Part model, mm, in its own coordinate system. A direction names the side the tool comes from. Coordinates: 2 decimals unless noted, no trailing zeros. Loops run counter-clockwise (first coordinate to the right, second up) from the corner with the lowest first, then second, coordinate; pieces in that order, holes last. Notation, with made-up numbers: (-25.75, -36.75) -> (29.25, -36.75) arc R12 cw to (29.25, -16.75) -> close; hole circle Ø2 at (-10, 1). An arc over 180 degrees is marked (long way). One line per question, with ' | ' between items. Start each with the question number.
1) 3-axis set-ups, long thin cutter, end or side, ignore diameter. For faces 1 (the face through (104.514, 32.972, -17.15)), 2 (the face through (-12, 0, 4)), 3 (the face through (4, -21, 21)): which of +Z, -Z, +X, -X, +Y, -Y reach the whole face in a straight line?
2) Cut at B-B (y = 0). List the corners of the cut face in (x, z).
3) Probe L1, parallel to X at y = 18.5, z = -14; L2, parallel to X at y = -44.5, z = -15; L3, parallel to Y at x = 5.5, z = 15.5. List the from-to ranges inside material, lowest first. Write a range as from..to.
4) Two-plate mould, pull along Z, no slides. Class faces 4 (the face through (-20, 0, 0)), 5 (the face through (4, -21, -21)), 6 (the face through (48.86, 2.64, 59.94)): released by +Z, released by -Z, zero draft, split by the parting line, or undercut.
5) Cut at A-A (z = 0). List the corners of the cut face in (x, y), plus the area to 3 significant figures.
6) Drop flat-ended pins along their axis: pin 1 (1.3 mm diameter, centred on y = -20.5, z = 21, fed in from -X); pin 2 (1.8 mm diameter, centred on x = -11.5, z = 4.5, fed in from +Y); pin 3 (1.6 mm diameter, centred on y = 0, z = 5, fed in from -X). Give the stop position or say it passes through.
7) Cut at C-C (x = 7.5). List the corners of the cut face in (y, z), plus the area to 3 significant figures.
from build123d import *

# Parameters (mm, degrees)
BOSS_EXTRUDE1_START = 4
SKETCH1_R           = 60
BOSS_EXTRUDE1_DEPTH = 91
SKETCH3_R           = 47.5
SKETCH3_R_2         = 2.25
BOSS_EXTRUDE2_DEPTH = 4
SKETCH4_R           = 6
BOSS_EXTRUDE3_DEPTH = 20
CUT_EXTRUDE1_START  = -15
CUT_EXTRUDE1_DEPTH  = 15


with BuildPart() as part:
    # Sketch1 → Boss-Extrude1 (new body)
    with BuildSketch(Plane(origin=(0, 0, 0), x_dir=(0, 0, -1), z_dir=(1, 0, 0)).offset(BOSS_EXTRUDE1_START)):
        Circle(SKETCH1_R)
    extrude(amount=BOSS_EXTRUDE1_DEPTH)

    # Sketch2 → Revolve1 (revolve)
    with BuildSketch(Plane.XY, mode=Mode.PRIVATE) as revolve1_sk:
        Polygon((95, 60), (105, 36), (105, 11), (109, 11), (109, 0), (105, 0), (95, 0), align=None)
    revolve(revolve1_sk.sketch.rotate(Axis((95, 0, 0), (-1, 0, 0)), 90), axis=Axis((95, 0, 0), (-1, 0, 0)))

    # Sketch3 → Boss-Extrude2 (add)
    with BuildSketch(Plane.ZY.offset(-4)):
        Circle(SKETCH3_R)
        with Locations((21.213203436, -21.213203436)):
            Circle(SKETCH3_R_2, mode=Mode.SUBTRACT)
        with Locations((-21.213203436, -21.213203436)):
            Circle(SKETCH3_R_2, mode=Mode.SUBTRACT)
        with Locations((-28.977774789, -7.764571353)):
            Circle(SKETCH3_R_2, mode=Mode.SUBTRACT)
        with Locations((-28.977774789, 7.764571353)):
            Circle(SKETCH3_R_2, mode=Mode.SUBTRACT)
        with Locations((-21.213203436, 21.213203436)):
            Circle(SKETCH3_R_2, mode=Mode.SUBTRACT)
        with Locations((-7.764571353, 28.977774789)):
            Circle(SKETCH3_R_2, mode=Mode.SUBTRACT)
        with Locations((7.764571353, 28.977774789)):
            Circle(SKETCH3_R_2, mode=Mode.SUBTRACT)
        with Locations((21.213203436, 21.213203436)):
            Circle(SKETCH3_R_2, mode=Mode.SUBTRACT)
        with Locations((28.977774789, 7.764571353)):
            Circle(SKETCH3_R_2, mode=Mode.SUBTRACT)
        with Locations((28.977774789, -7.764571353)):
            Circle(SKETCH3_R_2, mode=Mode.SUBTRACT)
    extrude(amount=BOSS_EXTRUDE2_DEPTH)

    # Sketch4 → Boss-Extrude3 (add)
    with BuildSketch(Plane.ZY):
        Circle(SKETCH4_R)
    extrude(amount=BOSS_EXTRUDE3_DEPTH)

    # Sketch5 → Cut-Extrude1 (cut)
    with BuildSketch(Plane.ZY.offset(20).offset(CUT_EXTRUDE1_START)):
        with BuildLine():
            Line((5.656854249, 2), (4, 2))
            Line((4, 2), (4, -2))
            Line((4, -2), (5.656854249, -2))
            ThreePointArc((5.656854249, -2), (6, 0), (5.656854249, 2))
        make_face()
    extrude(amount=CUT_EXTRUDE1_DEPTH, mode=Mode.SUBTRACT)


solid = part.part
Reported:
1) face 1: +X | face 2: +Z, -X | face 3: -X
2) outline: (-20, -6) -> (0, -6) -> (0, -47.5) -> (4, -47.5) -> (4, -60) -> (95, -60) -> (105, -36) -> (105, -11) -> (109, -11) -> (109, 11) -> (105, 11) -> (105, 36) -> (95, 60) -> (4, 60) -> (4, 47.5) -> (0, 47.5) -> (0, 6) -> (-5, 6) -> (-5, 4) -> (-20, 4) -> close
3) L1: x = 0..105 | L2: x = 0..100.43 | L3: y = -57.96..57.96
4) face 4: zero draft | face 5: undercut | face 6: split by the parting line
5) outline: (-20, -6) -> (0, -6) -> (0, -47.5) -> (4, -47.5) -> (4, -60) -> (95, -60) -> (105, -36) -> (105, -11) -> (109, -11) -> (109, 11) -> (105, 11) -> (105, 36) -> (95, 60) -> (4, 60) -> (4, 47.5) -> (0, 47.5) -> (0, 6) -> (-20, 6) -> close | area: 12,600 mm²
6) pin 1: stops at x = 4 | pin 2: stops at y = 4.8 | pin 3: stops at x = -5
7) outline: circle Ø120 at (0, 0) | area: 11,300 mm²
